from build123d import *

# Parameters (mm, degrees)
F0_R     = 2.7
F1_DEPTH = 30


with BuildPart() as f1:
    # F0 (on Top) → F1 (new body)
    with BuildSketch(Plane.XY):
        with BuildLine():
            ThreePointArc((-15.25, 11.75), (-12.775126, 12.775126), (-11.75, 15.25))
            ThreePointArc((-11.75, 15.25), (-15.25, 18.75), (-18.75, 15.25))
            ThreePointArc((-18.75, 15.25), (-18.435906, 13.800862), (-17.55, 12.611819))
            ThreePointArc((-17.55, 12.611819), (-16.478081, 11.972529), (-15.25, 11.75))
        make_face()
        with Locations((-15.25, 15.25)):
            Circle(F0_R, mode=Mode.SUBTRACT)
        with BuildLine():
            Line((-17.55, 10.5), (-15.25, 11.75))
            ThreePointArc((-15.25, 11.75), (-16.478081, 11.972529), (-17.55, 12.611819))
            Line((-17.55, 12.611819), (-17.55, 10.5))
        make_face()
        with BuildLine():
            ThreePointArc((-17.55, 12.611819), (-18.435906, 13.800862), (-18.75, 15.25))
            Line((-18.75, 15.25), (-18.75, -15.25))
            ThreePointArc((-18.75, -15.25), (-18.435906, -13.800862), (-17.55, -12.611819))
            Line((-17.55, -12.611819), (-17.55, -10.5))
            Line((-17.55, -10.5), (-17.55, 10.5))
            Line((-17.55, 10.5), (-17.55, 12.611819))
        make_face()
        with BuildLine():
            ThreePointArc((-17.55, -12.611819), (-18.435906, -13.800862), (-18.75, -15.25))
            ThreePointArc((-18.75, -15.25), (-17.724874, -17.724874), (-15.25, -18.75))
            ThreePointArc((-15.25, -18.75), (-13.800862, -18.435906), (-12.611819, -17.55))
            ThreePointArc((-12.611819, -17.55), (-11.972529, -16.478081), (-11.75, -15.25))
            ThreePointArc((-11.75, -15.25), (-12.775126, -12.775126), (-15.25, -11.75))
            ThreePointArc((-15.25, -11.75), (-16.478081, -11.972529), (-17.55, -12.611819))
        make_face()
        with Locations((-15.25, -15.25)):
            Circle(F0_R, mode=Mode.SUBTRACT)
        with BuildLine():
            Line((-17.55, -10.5), (-17.55, -12.611819))
            ThreePointArc((-17.55, -12.611819), (-16.478081, -11.972529), (-15.25, -11.75))
            Line((-15.25, -11.75), (-17.55, -10.5))
        make_face()
        with BuildLine():
            ThreePointArc((-11.75, -15.25), (-11.972529, -16.478081), (-12.611819, -17.55))
            Line((-12.611819, -17.55), (-10.5, -17.55))
            Line((-10.5, -17.55), (-11.75, -15.25))
        make_face()
        with BuildLine():
            ThreePointArc((-12.611819, -17.55), (-13.800862, -18.435906), (-15.25, -18.75))
            Line((-15.25, -18.75), (15.25, -18.75))
            ThreePointArc((15.25, -18.75), (13.800862, -18.435906), (12.611819, -17.55))
            Line((12.611819, -17.55), (10.5, -17.55))
            Line((10.5, -17.55), (-10.5, -17.55))
            Line((-10.5, -17.55), (-12.611819, -17.55))
        make_face()
        with BuildLine():
            Line((10.5, -17.55), (12.611819, -17.55))
            ThreePointArc((12.611819, -17.55), (11.972529, -16.478081), (11.75, -15.25))
            Line((11.75, -15.25), (10.5, -17.55))
        make_face()
        with BuildLine():
            ThreePointArc((12.611819, -17.55), (13.800862, -18.435906), (15.25, -18.75))
            ThreePointArc((15.25, -18.75), (17.724874, -17.724874), (18.75, -15.25))
            ThreePointArc((18.75, -15.25), (15.25, -11.75), (11.75, -15.25))
            ThreePointArc((11.75, -15.25), (11.972529, -16.478081), (12.611819, -17.55))
        make_face()
        with Locations((15.25, -15.25)):
            Circle(F0_R, mode=Mode.SUBTRACT)
    extrude(amount=F1_DEPTH)


solid = f1.part
The model under review builds one solid part; all positions refer to its coordinate system, in mm. A direction names the side the tool comes from. Give positions to 0.01 mm unless a question says otherwise; leave off trailing zeros. Loops run counter-clockwise (first coordinate to the right, second up) from the corner with the lowest first, then second, coordinate; pieces in that order, holes last. Notation, with made-up numbers: (-36.5, 65.5) -> (-0.5, 65.5) arc R29 cw to (-0.5, 98.5) -> close; hole circle Ø3 at (-25.5, 28). An arc over 180 degrees is marked (long way). Answer as a JSON object with one key per item and string values. Group by question number.
Q1. Take a section at B-B (x = 14.5). Write out the cut boundary in (y, z).
Q2. Insertion check: pin 1 (3 mm diameter, centred on x = -4, z = 4.5, fed in from +Y); pin 2 (7 mm diameter, centred on x = -15.25, y = 15.25, fed in from +Z); pin 3 (1 mm diameter, centred on y = -14, z = 25.5, fed in from +X); pin 4 (4 mm diameter, centred on y = 11, z = 16, fed in from +X). Each pin has a flat end and moves straight along its axis. Give the tip position at first contact, or say it passes through.
Q3. Take a section at D-D (x = -11). Write out the cut boundary in (y, z), plus the area to 3 significant figures.
Q4. Draft analysis for pull direction Y (two halves, no side actions). For faces 4 (the cylindrical face through (-13.798, -12.973, 14.79)), 5 (the flat face through (-18.75, 0, 15)), 6 (the flat face through (11.134, -16.384, 14.79)), state which applies: pulls with the +Y half, pulls with the -Y half, needs draft (parallel to the pull), parting line crosses it, or undercut.
Q5. Tool access review of faces 1 (the cylindrical face through (-12.75, -12.8, 14.79)), 2 (the flat face through (-16.416, 11.116, 14.79)), 3 (the flat face through (-11.116, -16.416, 14.79)): name each direction out of +Z, -Z, +X, -X, +Y, -Y from which nothing blocks a thin tool from reaching the whole face with its end or side.
Q6. Take a section at A-A (z = 27.25). Write out the cut boundary in (x, y).
Q7. Wall thickness on line 1 along Y through (x, z) = (-15.25, 16.5); line 2 along Y through (x, z) = (15.25, 20); line 3 along X through (y, z) = (15, 8): over which ranges is each line inside the solid? List them lowest first.
Q8. Take a section at C-C (y = -16). Write out the cut boundary in (x, z), plus the area to 3 significant figures.
Answer below:
{
 "1": {"outline": "(-18.75, 0) -> (-17.84, 0) -> (-17.84, 30) -> (-18.75, 30) -> close; (-12.66, 0) -> (-11.83, 0) -> (-11.83, 30) -> (-12.66, 30) -> close"},
 "2": {"pin 1": "stops at y = -17.55", "pin 2": "stops at z = 30", "pin 3": "stops at x = 18.67", "pin 4": "stops at x = -12.57"},
 "3": {"outline": "(-18.75, 0) -> (-16.63, 0) -> (-16.63, 30) -> (-18.75, 30) -> close", "area": "63.6 mm2"},
 "4": {"face 4": "undercut", "face 5": "needs draft", "face 6": "pulls with the +Y half"},
 "5": {"face 1": "+Z, -Z", "face 2": "+Z, -Z, +X", "face 3": "+Z, -Z, +Y"},
 "6": {"outline": "(-18.75, -15.25) arc R3.5 ccw to (-15.25, -18.75) -> (15.25, -18.75) arc R3.5 ccw (long way) to (11.75, -15.25) -> (10.5, -17.55) -> (-10.5, -17.55) -> (-11.75, -15.25) arc R3.5 ccw to (-15.25, -11.75) -> (-17.55, -10.5) -> (-17.55, 10.5) -> (-15.25, 11.75) arc R3.5 ccw (long way) to (-18.75, 15.25) -> close; hole circle Ø5.4 at (-15.25, -15.25); hole circle Ø5.4 at (-15.25, 15.25); hole circle Ø5.4 at (15.25, -15.25)"},
 "7": {"line 1": "y = -18.75 to -17.95, -12.55 to -11.75, 11.75 to 12.55, 17.95 to 18.75", "line 2": "y = -18.75 to -17.95, -12.55 to -11.75", "line 3": "x = -18.75 to -17.94, -12.56 to -11.76"},
 "8": {"outline": "(-18.67, 0) -> (-17.84, 0) -> (-17.84, 30) -> (-18.67, 30) -> close; (-12.66, 0) -> (-11.34, 0) -> (-11.34, 30) -> (-12.66, 30) -> close; (11.34, 0) -> (12.66, 0) -> (12.66, 30) -> (11.34, 30) -> close; (17.84, 0) -> (18.67, 0) -> (18.67, 30) -> (17.84, 30) -> close", "area": "128 mm2"}
}
